The listing builds one solid part. Answer for the finished solid, in the listing's coordinates (mm). A direction names the side the tool comes from. Give positions to 0.01 mm unless a question says otherwise; leave off trailing zeros. Order: outer loops, then holes, each group sorted by start corner. A loop starts at its lowest first (then second) coordinate and runs counter-clockwise, first axis right, second up. Notation, with made-up numbers: (37.25, 71) - (95.25, 71) arc R16 ccw to (95.25, 102) - close; hole circle Ø2 at (12, 6). An arc over 180 degrees is marked (long way). Use a Markdown table: item, result. Add a question column.
1) Find section B-B, the plane x = -21. Determine the outline of the cut face in (y, z), plus the area to 3 significant figures.
2) Find section C-C, the plane z = 16. Determine the outline of the cut face in (x, y).
3) Find section A-A, the plane y = -11.25. Determine the outline of the cut face in (x, z).
4) Straight lines are drawn through the part: line 1 (Z direction, x = 7, y = -18.75); line 2 (X direction, y = -8.5, z = 76.5). For each, find the intervals that lie inside material, in ascending order.
5) Flat-ended cylindrical pins translate along their axes: pin 1 (7.5 mm diameter, centred on y = -8.5, z = 20.5, fed in from -X); pin 2 (7.5 mm diameter, centred on x = -41.5, y = -9.5, fed in from -Z); pin 3 (1.5 mm diameter, centred on x = -5, y = -10, fed in from +Z). Find the tip coordinate at first contact, or state that the pin passes through.
6) For faces 1 (the face through (-4, -13, 0)), 2 (the face through (-31, -13, 49.762)), 3 (the face through (-32, -13, 39.079)), 4 (the face through (0, -13, 19)), 5 (the face through (0, -13, 69)), determine the directions among +Z, -Z, +X, -X, +Y, -Y from which every point of the face is accessible in a straight line to the end or side of a thin tool.
from build123d import *

# Parameters (mm, degrees)
F0_W     = 45.9087826312
F0_H     = 10.6835663319
F0_W_2   = 8.5728019476
F0_W_3   = 36.0127463937
F1_DEPTH = 25.4
F0_H_2   = 39.0786156058
F2_DEPTH = 25.4


# Not quite as in the source:
# - a feature names something its author has since deleted; it is built from what else it names


with BuildPart() as f1:
    # F0 (on Front) → F1 (new body)
    with BuildSketch(Plane.XZ):
        with Locations((-31.5271932632, 44.4203987718)):
            Rectangle(F0_W, F0_H)
        with Locations((-4.2864009738, 44.4203987718)):
            Rectangle(F0_W_2, F0_H)
        with Locations((18.0063731968, 44.4203987718)):
            Rectangle(F0_W_3, F0_H)
    extrude(amount=F1_DEPTH)

    # F0 (on Front) → F2 (join)
    with BuildSketch(Plane.XZ):
        with Locations((-4.2864009738, 19.5393078029)):
            Rectangle(F0_W_2, F0_H_2)
        with Locations((-4.2864009738, 44.4203987718)):
            Rectangle(F0_W_2, F0_H)
        Polygon((-8.5728019476, 87.886022841), (-8.5728019476, 49.7621819377), (0, 49.7621819377), (0, 88.8135335598), align=None)
    extrude(amount=F2_DEPTH)


solid = f1.part
The answers:
| question | item | result |
|---|---|---|
| 1 | outline | (-25.4, 39.08) - (0, 39.08) - (0, 49.76) - (-25.4, 49.76) - close |
| 1 | area | 271 mm2 |
| 2 | outline | (-8.57, -25.4) - (0, -25.4) - (0, 0) - (-8.57, 0) - close |
| 3 | outline | (-54.48, 39.08) - (-8.57, 39.08) - (-8.57, 0) - (0, 0) - (0, 39.08) - (36.01, 39.08) - (36.01, 49.76) - (0, 49.76) - (0, 88.81) - (-8.57, 87.89) - (-8.57, 49.76) - (-54.48, 49.76) - close |
| 4 | line 1 | 39.08 to 49.76 |
| 4 | line 2 | -8.57 to 0 |
| 5 | pin 1 | x = -8.57 |
| 5 | pin 2 | z = 39.08 |
| 5 | pin 3 | z = 88.35 |
| 6 | face 1 | -Z, +X, -X, +Y, -Y |
| 6 | face 2 | +Z, -X, +Y, -Y |
| 6 | face 3 | -Z, -X, +Y, -Y |
| 6 | face 4 | -Z, +X, +Y, -Y |
| 6 | face 5 | +Z, +X, +Y, -Y |
